from build123d import *

# Parameters (mm, degrees)
BASPROSKE_W        = 3
BASPROSKE_H        = 9
TOOTHCUT_DEPTH     = 14.076696831
TEETHCUTS_COUNT    = 18
TEETHCUTS_ANGLE    = 340
CUT_EXTRUDE1_DEPTH = 14.007462246


with BuildPart() as part:
    # BasProSke → Base-Revolve (revolve)
    with BuildSketch(Plane(origin=(0, 0, 0), x_dir=(1, 0, 0), z_dir=(0, 1, 0)), mode=Mode.PRIVATE) as base_revolve_sk:
        with Locations((1.5, 4.5)):
            Rectangle(BASPROSKE_W, BASPROSKE_H)
    revolve(base_revolve_sk.sketch.rotate(Axis((-10, 0, 0), (1, 0, 0)), 180), axis=Axis((-10, 0, 0), (1, 0, 0)))

    # TooCutSke → ToothCut (cut, through all)
    with BuildSketch(Plane(origin=(0, 0, 0), x_dir=(0, 0, -1), z_dir=(1, 0, 0))):
        with BuildLine():
            ThreePointArc((0.45926649, 6.958861278), (0, 6.974), (-0.45926649, 6.958861278))
            ThreePointArc((-0.45926649, 6.958861278), (-0.743858876, 8.01799277), (-1.365479267, 8.921508366))
            ThreePointArc((-1.365479267, 8.921508366), (0, 9.0254), (1.365479267, 8.921508366))
            ThreePointArc((1.365479267, 8.921508366), (0.743858876, 8.01799277), (0.45926649, 6.958861278))
        make_face()
    toothcut = extrude(amount=TOOTHCUT_DEPTH, mode=Mode.SUBTRACT)

    # TeethCuts: ToothCut ×18 about axis
    teethcuts_axis = Axis((-10, 0, 0), (1, 0, 0))
    for i in range(1, TEETHCUTS_COUNT):
        add(toothcut.rotate(teethcuts_axis, i * TEETHCUTS_ANGLE / (TEETHCUTS_COUNT - 1)), mode=Mode.SUBTRACT)

    # Sketch1 → Cut-Extrude1 (cut, through all)
    with BuildSketch(Plane(origin=(3, 0, 0), x_dir=(0, 0, -1), z_dir=(1, 0, 0))):
        Polygon((0, 3.960622847), (-3.43, 1.980311423), (-3.43, -1.980311423), (0, -3.960622847), (3.43, -1.980311423), (3.43, 1.980311423), align=None)
    extrude(amount=-CUT_EXTRUDE1_DEPTH, mode=Mode.SUBTRACT)


solid = part.part
Can you work these out from the model? Positions are in its coordinate system, mm. A direction names the side the tool comes from. Give positions to 0.01 mm unless a question says otherwise; leave off trailing zeros. Write each loop counter-clockwise with the first axis right and the second up, starting at its lowest first coordinate (ties: lowest second). Pieces come first, ordered by that corner, then holes. Notation, with made-up numbers: (62, -35.75) -> (87, -35.75) arc R32 cw to (87, 0.25) -> close; hole circle Ø4 at (-13, -9.75). An arc over 180 degrees is marked (long way). Answer as a JSON object with one key per item and string values. Group by question number.
Item 1: Suppose I cut it at B-B (y = 5.25). Please give me the cut outline in (x, z).
Item 2: Suppose I cut it at C-C (z = 1). Please give me the cut outline in (x, y), plus the area to 3 significant figures.
Item 3: For faces 4 (the face through (1.479, 6.62, 4.584)), 5 (the face through (1.48, 4.65, 6.57)), 6 (the face through (1.48, 7.99, 0.73)), which set-ups out of +Z, -Z, +X, -X, +Y, -Y let a thin tool reach every point of the face, with its end or its side?
Item 4: Suppose I cut it at A-A (z = 8). Please give me the cut outline in (x, y), plus the area to 3 significant figures.
Item 5: Please list where these lines run through material, in increasing order: line 1 (Y direction, x = 1.05, z = -7.5); line 2 (Z direction, x = 1.4, y = 7.25); line 3 (Z direction, x = 1.2, y = 6.75). Write a range as [from, to].
Item 6: I'm going to push flat-ended pins straight in: P1, Ø1.5, axis at x = 2, z = 0.5, coming from the +Y side; P2, Ø1, axis at x = 2.5, z = 6.5, coming from the +Y side. Where does each tip first touch, or does it pass through?
Item 7: We'd pull the mould along Y, two halves only. Please class faces 1 (the face through (1.479, 5.664, -5.723)), 2 (the face through (1.479, 1.217, 6.867)), 3 (the face through (1.48, -7.99, -0.73)): +Y half, -Y half, draft (parallel to the pull), parting line (faces both ways), or undercut.
Findings:
{
 "1": {"outline": "(0, -6.9) -> (3, -6.9) -> (3, -5.06) -> (0, -5.06) -> close; (0, -4.59) -> (3, -4.59) -> (3, 4.59) -> (0, 4.59) -> close; (0, 5.06) -> (3, 5.06) -> (3, 6.9) -> (0, 6.9) -> close"},
 "2": {"outline": "(0, -8.47) -> (3, -8.47) -> (3, -3.38) -> (0, -3.38) -> close; (0, 3.38) -> (3, 3.38) -> (3, 8.47) -> (0, 8.47) -> close", "area": "30.5 mm²"},
 "3": {"face 4": "+X, -X", "face 5": "+Z, +X, -X", "face 6": "+X, -X, +Y"},
 "4": {"outline": "(0, -3.35) -> (3, -3.35) -> (3, -2.3) -> (0, -2.3) -> close; (0, -0.67) -> (3, -0.67) -> (3, 0.67) -> (0, 0.67) -> close; (0, 2.3) -> (3, 2.3) -> (3, 3.35) -> (0, 3.35) -> close", "area": "10.3 mm²"},
 "5": {"line 1": "y = [-3.38, -1.96], [-0.75, 0.75], [1.96, 3.38]", "line 2": "z = [-4.69, -3.41], [-2.04, -0.5], [0.5, 2.04], [3.41, 4.69]", "line 3": "z = [-4.62, -3.02], [-1.96, 1.96], [3.02, 4.62]"},
 "6": {"P1": "stops at y = 8.8", "P2": "stops at y = 5.95"},
 "7": {"face 1": "+Y half", "face 2": "undercut", "face 3": "-Y half"}
}
